Could you check a few things on this drawing? It's one solid part, dimensions in mm from its lowest x, y, z. Give positions to 0.01 mm unless a question says otherwise; leave off trailing zeros. Order: outer loops, then holes, each group sorted by start corner. A loop starts at its lowest first (then second) coordinate and runs counter-clockwise, first axis right, second up. Notation, with made-up numbers: (35.5, 75.5) -> (88.5, 75.5) arc R32 ccw to (88.5, 103.5) -> close; hole circle Ø10 at (-17.5, 1.25). An arc over 180 degrees is marked (long way). Use one line per item in the form item = value. Start each with the question number.
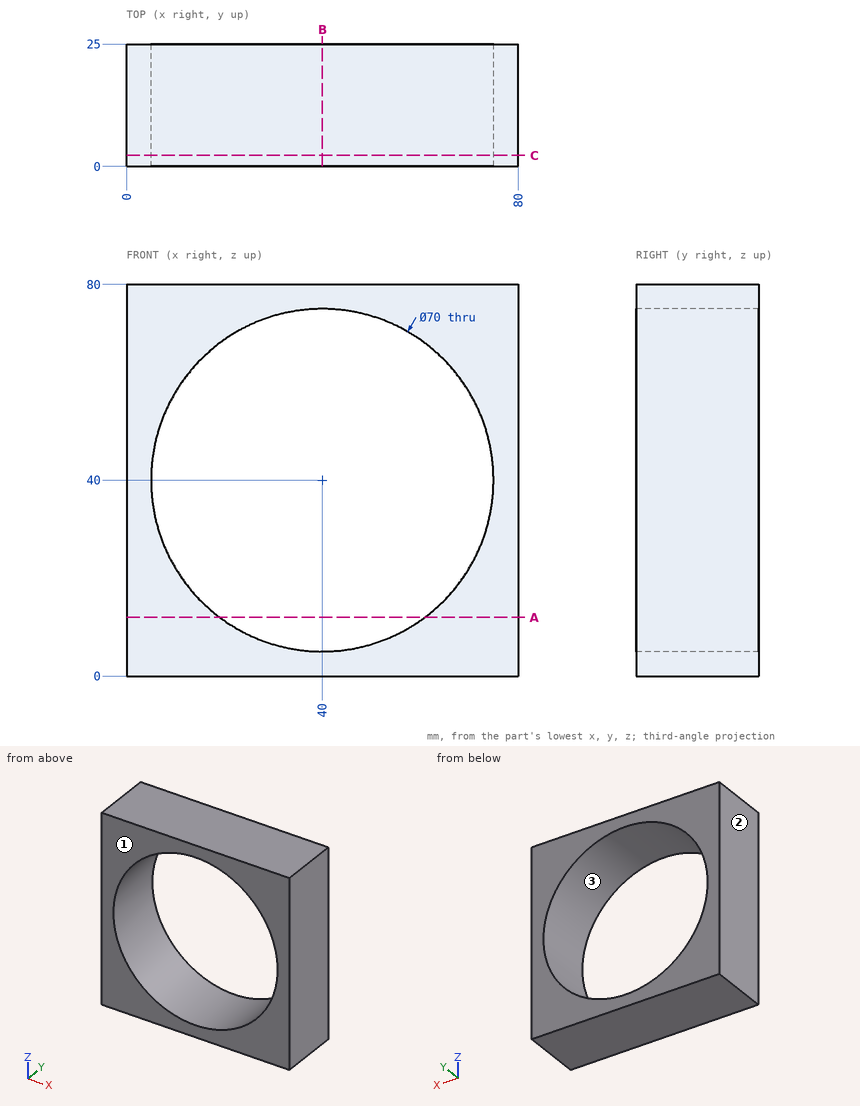
(1) Please list where these lines run through material, in increasing order: probe 1 along Z at (x, y) = (40, 15.5); probe 2 along Z at (x, y) = (49.5, 17.5); probe 3 along X at (y, z) = (5.25, 57).
(2) Imagine slicing it at C-C (y = 2.25). Write out the boundary of the cut face in (x, z).
(3) We'd pull the mould along X, two halves only. Please class the marked faces 1, 2 and 3: pulls with the +X half, pulls with the -X half, needs draft (parallel to the pull), parting line crosses it, or undercut.
(4) Imagine slicing it at B-B (x = 40). Write out the boundary of the cut face in (y, z), plus the area to 3 significant figures.
(5) Imagine slicing it at A-A (z = 12). Write out the boundary of the cut face in (x, y).
Calculated:
q1.probe_1 = 0 to 5, 75 to 80
q1.probe_2 = 0 to 6.31, 73.69 to 80
q1.probe_3 = 0 to 9.41, 70.59 to 80
q2.outline = (0, 0) -> (80, 0) -> (80, 80) -> (0, 80) -> close; hole circle Ø70 at (40, 40)
q3.face_1 = needs draft
q3.face_2 = pulls with the -X half
q3.face_3 = undercut
q4.outline = (0, 0) -> (25, 0) -> (25, 5) -> (0, 5) -> close; (0, 75) -> (25, 75) -> (25, 80) -> (0, 80) -> close
q4.area = 250 mm2
q5.outline = (0, 0) -> (19, 0) -> (19, 25) -> (0, 25) -> close; (61, 0) -> (80, 0) -> (80, 25) -> (61, 25) -> close
